from build123d import *

# Parameters (mm, degrees)
SKETCH_3_R             = 3.375
SKETCH_3_R_2           = 1.55
EXTRUDE_1_DEPTH        = 4.5
FILLET_1_R             = 5
CUT_EXTRUDE_2_REACH    = 155.806
FILLET_3_R             = 3
EXTRUDE_4428_DEPTH     = 4.5
SKETCH_7_R             = 5.5
CUT_EXTRUDE_4738_DEPTH = 154.806186932
FILLET_1_2_R           = 3


with BuildPart() as part:
    # 草图3 → 凸台-拉伸1 (new body)
    with BuildSketch(Plane(origin=(0, 0, 0), x_dir=(1, 0, 0), z_dir=(0, 1, 0))):
        with BuildLine():
            Line((41.131907973, -24.012757507), (94.694386062, -62.928175745))
            Line((94.694386062, -62.928175745), (100.131399646, -55.444768547))
            Line((100.131399646, -55.444768547), (122.783875489, -71.902755611))
            Line((122.783875489, -71.902755611), (106.325888424, -94.555231453))
            Line((106.325888424, -94.555231453), (95.372658906, -86.597244389))
            Line((95.372658906, -86.597244389), (56.836706291, -86.597244389))
            Line((56.836706291, -86.597244389), (42.973762785, -95.097244389))
            Line((42.973762785, -95.097244389), (30, -95.097244389))
            Line((30, -95.097244389), (30, -86.597244389))
            Line((30, -86.597244389), (42.973762785, -86.597244389))
            Line((42.973762785, -86.597244389), (56.836706291, -78.097244389))
            Line((56.836706291, -78.097244389), (83.673412582, -78.097244389))
            Line((83.673412582, -78.097244389), (89.110426166, -70.613837191))
            Line((89.110426166, -70.613837191), (35.547948076, -31.698418954))
            ThreePointArc((35.547948076, -31.698418954), (34.497097301, -25.063608282), (41.131907973, -24.012757507))
        make_face()
        with Locations(Location((103.228644035, -75, 0), (0, 0, 270))):
            Circle(SKETCH_3_R, mode=Mode.SUBTRACT)
        with Locations(Location((44.044221455, -32, 0), (0, 0, 270))):
            Circle(SKETCH_3_R_2, mode=Mode.SUBTRACT)
        with Locations(Location((60.224561343, -43.755705046, 0), (0, 0, 270))):
            Circle(SKETCH_3_R_2, mode=Mode.SUBTRACT)
        with Locations(Location((34.5, -90.847244389, 0), (0, 0, 270))):
            Circle(SKETCH_3_R_2, mode=Mode.SUBTRACT)
        with BuildLine():
            Line((110.640755254, -72.256715968), (112.616131935, -71.943847038))
            ThreePointArc((112.616131935, -71.943847038), (114.389522284, -73.232290545), (113.101078777, -75.005680894))
            Line((113.101078777, -75.005680894), (111.125702096, -75.318549824))
            ThreePointArc((111.125702096, -75.318549824), (109.352311747, -74.030106317), (110.640755254, -72.256715968))
        make_face(mode=Mode.SUBTRACT)
        with BuildLine():
            Line((103.547193859, -67.10294194), (103.234324929, -65.127565258))
            ThreePointArc((103.234324929, -65.127565258), (101.46093458, -63.839121751), (100.172491073, -65.6125121))
            Line((100.172491073, -65.6125121), (100.485360003, -67.587888781))
            ThreePointArc((100.485360003, -67.587888781), (102.258750352, -68.876332288), (103.547193859, -67.10294194))
        make_face(mode=Mode.SUBTRACT)
        with BuildLine():
            Line((95.816532817, -77.743284032), (93.841156135, -78.056152962))
            ThreePointArc((93.841156135, -78.056152962), (92.067765787, -76.767709455), (93.356209294, -74.994319106))
            Line((93.356209294, -74.994319106), (95.331585975, -74.681450176))
            ThreePointArc((95.331585975, -74.681450176), (97.104976324, -75.969893683), (95.816532817, -77.743284032))
        make_face(mode=Mode.SUBTRACT)
        with BuildLine():
            Line((102.910094211, -82.89705806), (103.222963142, -84.872434742))
            ThreePointArc((103.222963142, -84.872434742), (104.99635349, -86.160878249), (106.284796997, -84.3874879))
            Line((106.284796997, -84.3874879), (105.971928067, -82.412111219))
            ThreePointArc((105.971928067, -82.412111219), (104.198537719, -81.123667712), (102.910094211, -82.89705806))
        make_face(mode=Mode.SUBTRACT)
    extrude(amount=EXTRUDE_1_DEPTH)

    # Fillet 1
    fillet_1_edges = [part.edges().sort_by_distance(p)[0] for p in [
        (83.673412582, 2.25, 78.097244389),
        (89.110426166, 2.25, 70.613837191),
        (100.131399646, 2.25, 55.444768547),
        (122.783875489, 2.25, 71.902755611),
        (106.325888424, 2.25, 94.555231453),
    ]]
    fillet(fillet_1_edges, radius=FILLET_1_R)

    # 草图4 → 圆弧-美观2 (cut, up to next)
    with BuildSketch(Plane(origin=(0, 4.5, 0), x_dir=(1, 0, 0), z_dir=(0, 1, 0)), mode=Mode.PRIVATE) as cut_extrude_2_sk1:
        with BuildLine():
            ThreePointArc((118.738790517, -68.963829349), (109.994899962, -65.687047674), (104.176484618, -58.383694808))
            Line((104.176484618, -58.383694808), (118.738790517, -68.963829349))
        make_face()
    cut_extrude_2_tool1 = extrude(cut_extrude_2_sk1.sketch, amount=-CUT_EXTRUDE_2_REACH, mode=Mode.PRIVATE) & part.part
    # 草图4 → 圆弧-美观2 (cut, up to next)
    with BuildSketch(Plane(origin=(0, 4.5, 0), x_dir=(1, 0, 0), z_dir=(0, 1, 0)), mode=Mode.PRIVATE) as cut_extrude_2_sk2:
        with BuildLine():
            ThreePointArc((119.844949227, -75.947840583), (112.204348353, -81.521230905), (109.264814686, -90.510146481))
            Line((109.264814686, -90.510146481), (119.844949227, -75.947840583))
        make_face()
    cut_extrude_2_tool2 = extrude(cut_extrude_2_sk2.sketch, amount=-CUT_EXTRUDE_2_REACH, mode=Mode.PRIVATE) & part.part
    add(cut_extrude_2_tool1.solids().sort_by_distance((110.868828, 4.5, 64.48419))[0], mode=Mode.SUBTRACT)
    add(cut_extrude_2_tool2.solids().sort_by_distance((113.606622, 4.5, 82.540042))[0], mode=Mode.SUBTRACT)

    # 圆角-美观3
    fillet_3_edges = [part.edges().sort_by_distance(p)[0] for p in [
        (119.844949227, 2.25, 75.947840583),
        (109.264814686, 2.25, 90.510146481),
        (118.738790517, 2.25, 68.963829349),
        (104.176484618, 2.25, 58.383694808),
        (95.372658906, 2.25, 86.597244389),
        (30, 2.25, 95.097244389),
        (30, 2.25, 86.597244389),
        (94.694386062, 2.25, 62.928175745),
    ]]
    fillet(fillet_3_edges, radius=FILLET_3_R)

    # 草图5 → Extrude 4428 (add)
    with BuildSketch(Plane(origin=(0, 0, 0), x_dir=(1, 0, 0), z_dir=(0, 1, 0))):
        with BuildLine():
            Line((34, -4.25), (27.002484736, -4.25))
            ThreePointArc((27.002484736, -4.25), (27.592720055, -7.98965282), (28.516665153, -11.661124786))
            ThreePointArc((28.516665153, -11.661124786), (28.909483525, -13.772484831), (28.842431122, -15.919028912))
            ThreePointArc((28.842431122, -15.919028912), (30.008908493, -24.737793116), (35.547948076, -31.698418954))
            ThreePointArc((35.547948076, -31.698418954), (34.497097301, -25.063608282), (41.131907973, -24.012757507))
            Line((41.131907973, -24.012757507), (54.395000648, -33.648958388))
            ThreePointArc((54.395000648, -33.648958388), (41.285942601, -17.872891342), (37.310903062, 2.249999975))
            Line((37.310903062, 2.249999975), (34, 2.249999975))
            Line((34, 2.249999975), (34, -4.25))
        make_face()
    extrude(amount=EXTRUDE_4428_DEPTH)

    # 草图7 → Cut-Extrude 4738 (cut, through all)
    with BuildSketch(Plane(origin=(0, 0, 0), x_dir=(1, 0, 0), z_dir=(0, 1, 0))):
        with Locations((28, -28)):
            Circle(SKETCH_7_R)
    extrude(amount=CUT_EXTRUDE_4738_DEPTH, mode=Mode.SUBTRACT)

    # Fillet 1 2
    fillet_1_2_edges = [part.edges().sort_by_distance(p)[0] for p in [
        (33.239893047, 2.25, 29.671382916),
        (29.281526942, 2.25, 22.651384413),
    ]]
    fillet(fillet_1_2_edges, radius=FILLET_1_2_R)


solid = part.part
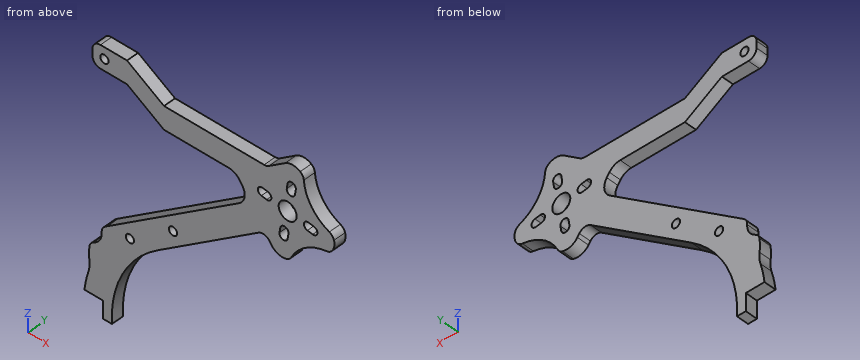
The listing builds one solid part. Answer for the finished solid, in the listing's coordinates (mm). Give positions to 0.01 mm unless a question says otherwise; leave off trailing zeros. Loops run counter-clockwise (first coordinate to the right, second up) from the corner with the lowest first, then second, coordinate; pieces in that order, holes last.
Item 1: Each of these flat-tipped pins is pushed along its axis until it touches: pin 1 Ø1 at (x, z) = (94, 77) entering from -Y; pin 2 Ø1.3 at (x, y) = (31, 2.5) entering from -Z; pin 3 Ø2 at (y, z) = (3, 91) entering from -X; pin 4 Ø1.3 at (x, y) = (67, 3) entering from -Z. Where does it stop, or does it pass through?
Derived:
pin 1: passes through
pin 2: stops at z = 4.25
pin 3: stops at x = 30
pin 4: stops at z = 42.33
Item 2: A cutting plane is placed at C-C (y = 0.7). Give the number of separate pieces and of enclosed holes in the cut face, then the cut area to 3 significant figures.
Derived:
separate pieces: 1
enclosed holes: 8
area: 2,030 mm2
Item 3: Find the intervals of material crossed by line 1 along X through (y, z) = (0.5, 74); line 2 along Z through (x, y) = (43.5, 2.4); line 3 along Z through (x, y) = (90, 3.45), in increasing order.
Derived:
line 1: x = 86.58 to 100.01, 106.45 to 109.35, 114.32 to 120.7
line 2: z = 21.93 to 30.55, 33.45 to 37.48, 86.27 to 94.77
line 3: z = 59.52 to 86.6
Item 4: A cutting plane is placed at B-B (x = 78). Give the vertices of the cut face in (y, z), then the cut area to 3 significant figures.
Derived:
outline: (0, 50.8) - (4.5, 50.8) - (4.5, 62.54) - (0, 62.54) - close; (0, 78.1) - (4.5, 78.1) - (4.5, 86.6) - (0, 86.6) - close
area: 91.1 mm2
Item 5: A cutting plane is placed at A-A (x = 41). Give the vertices of the cut face in (y, z), then the cut area to 3 significant figures.
Derived:
outline: (0, 17.26) - (4.5, 17.26) - (4.5, 35.66) - (0, 35.66) - close; (0, 86.6) - (4.5, 86.6) - (4.5, 95.1) - (0, 95.1) - close
area: 121 mm2
